Geometry: final body of the model. Coordinates: model frame, mm. Face numbers are marked on the shaded views. A direction names the side the tool comes from. Give positions to 0.01 mm unless a question says otherwise; leave off trailing zeros. Order: outer loops, then holes, each group sorted by start corner. A loop starts at its lowest first (then second) coordinate and runs counter-clockwise, first axis right, second up. Notation, with made-up numbers: (59.25, 47.25) -> (89.25, 47.25) arc R25 cw to (89.25, 76.25) -> close; hole circle Ø6 at (36, 80.5). An arc over 180 degrees is marked (long way). Answer in a Markdown table with one row per item. Add a question column.
Q1. Contact query for a flat-ended pin moving along its axis: P1, Ø1, axis at x = -2.5, y = 6, coming from the -Z side. Output: stop coordinate, or through.
Q2. Cut plane B-B on y = 5.5. Return the cut outline in (x, z), and give its area (3 significant figures).
Q3. Set-up query: the marked faces 1, 2 and 3. Return all of +Z, -Z, +X, -X, +Y, -Y with unobstructed straight access to the full face (end or side cutting, diameter ignored); none if empty.
Q4. Pull-direction query (X, two-part tool) for the marked faces 4, 5 and 6; classes: +X half, -X half, draft (parallel to the pull), parting line (faces both ways), or undercut.
Q5. Line query: line 1 along X through (y, z) = (6.5, 2); line 2 along Y through (x, z) = (-10.25, 1.25); line 3 along Z through (x, y) = (-9.25, 5.5). Output: solid intervals per line, ascending. Write a range as from..to.
Q6. Cut plane C-C on x = -7.25. Return the cut outline in (y, z), and give its area (3 significant figures).
Q7. Cut plane A-A on z = 4. Return the cut outline in (x, y).
Autodesk Inventor part; units mm, degrees
ref_plane "YZ Plane" through (0, 0, 0) normal (1, 0, 0) x (0, 1, 0)
ref_plane "XZ Plane" through (0, 0, 0) normal (0, 1, 0) x (-1, 0, 0)
ref_plane "XY Plane" through (0, 0, 0) normal (0, 0, 1) x (1, 0, 0)
sketch "Sketch5" plane through (0, 0, 0) normal (0, 0, 1) x (1, 0, 0)
  line L0 (0, 0) -> (-13.9, 0)
  line L1 (-13.9, 0) -> (-13.9, 9)
  line L2 (-13.9, 9) -> (0, 9)
  line L3 (0, 9) -> (0, 0)
  line L4 (-2, 2) -> (-11.9, 2)
  line L5 (-11.9, 2) -> (-11.9, 7)
  line L6 (-11.9, 7) -> (-2, 7)
  line L7 (-2, 7) -> (-2, 2)
  dimension "d67" = 13.9
  dimension "d68" = 9
  dimension "d69" = 9.9
  dimension "d70" = 5
extrude "Extrusion8" add sketch "Sketch5" along normal blind 12 contours L0 L1 L2 L3 | L4 L5 L6 L7
sketch "Sketch6" plane through (0, 0, 12) normal (0, 0, 1) x (1, 0, 0)
  line L0 (-1.7, 2) -> (-12.2, 2)
  line L1 (-12.2, 2) -> (-12.2, 7)
  line L2 (-12.2, 7) -> (-1.7, 7)
  line L3 (-1.7, 7) -> (-1.7, 2)
  point P0 (0, 0)
  dimension "d85" = 10.5
  dimension "d86" = 5
sketch "Sketch7" plane through (0, 0, 0) normal (0, 0, -1) x (-1, 0, 0)
  line L0 (1.7, 2) -> (12.2, 2)
  line L1 (12.2, 2) -> (12.2, 7)
  line L2 (12.2, 7) -> (1.7, 7)
  line L3 (1.7, 7) -> (1.7, 2)
  point P0 (0, 0)
  dimension "d83" = 10.5
  dimension "d84" = 5
extrude "Extrusion12" cut sketch "Sketch6" against normal blind 5
extrude "Extrusion13" cut sketch "Sketch7" against normal blind 5
properties part number "Cube_Holder_SB_V1_(71mm)"
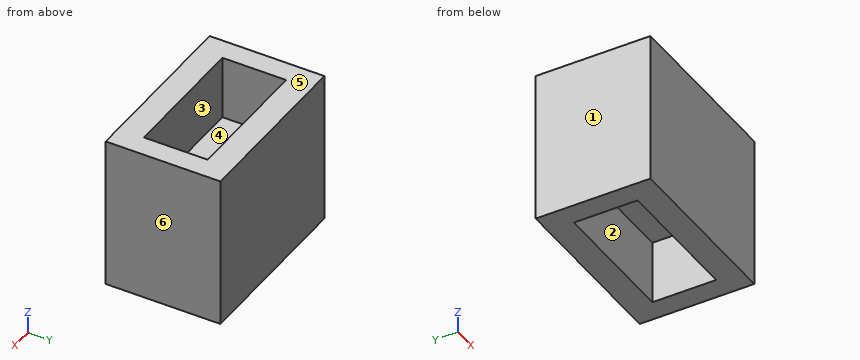
Completed:
| question | item | result |
|---|---|---|
| 1 | P1 | stops at z = 5 |
| 2 | outline | (-13.9, 0) -> (-12.2, 0) -> (-12.2, 5) -> (-1.7, 5) -> (-1.7, 0) -> (0, 0) -> (0, 12) -> (-1.7, 12) -> (-1.7, 7) -> (-12.2, 7) -> (-12.2, 12) -> (-13.9, 12) -> close |
| 2 | area | 61.8 mm² |
| 3 | face 1 | +Z, -Z, -X, +Y, -Y |
| 3 | face 2 | -Z |
| 3 | face 3 | +Z |
| 4 | face 4 | undercut |
| 4 | face 5 | draft |
| 4 | face 6 | +X half |
| 5 | line 1 | x = -13.9..-12.2, -1.7..0 |
| 5 | line 2 | y = 0..2, 7..9 |
| 5 | line 3 | z = 5..7 |
| 6 | outline | (0, 0) -> (2, 0) -> (2, 5) -> (7, 5) -> (7, 0) -> (9, 0) -> (9, 12) -> (7, 12) -> (7, 7) -> (2, 7) -> (2, 12) -> (0, 12) -> close |
| 6 | area | 58.0 mm² |
| 7 | outline | (-13.9, 0) -> (0, 0) -> (0, 9) -> (-13.9, 9) -> close; hole (-12.2, 2) -> (-1.7, 2) -> (-1.7, 7) -> (-12.2, 7) -> close |
